Autodesk Inventor part; units mm, degrees
ref_plane "XZ Plane" through (0, 0, 0) normal (0, 1, 0) x (-1, 0, 0)
ref_plane "XY Plane" through (0, 0, 0) normal (0, 0, 1) x (1, 0, 0)
sketch "Sketch2" plane through (0, 0, 0) normal (0, 1, 0) x (-1, 0, 0)
  line L0 (35.5, -4) -> (35.5, 25)
  line L1 (35.5, 25) -> (31.5, 25)
  line L2 (31.5, 25) -> (31.5, 0)
  line L3 (31.5, 0) -> (-31.5, 0)
  line L4 (-31.5, 0) -> (-31.5, 25)
  line L5 (-31.5, 25) -> (-35.5, 25)
  line L6 (-35.5, 25) -> (-35.5, -4)
  line L7 (-35.5, -4) -> (35.5, -4)
  line L8 (0, -9.8) -> (0, 30.8) construction
  line L9 (-49.7, 0) -> (49.7, 0) construction
  point P0 (0, 0)
  dimension "d0" = 4
  dimension "d1" = 25
  dimension "d2" = 71
  dimension "d3" = 4
extrude "Extrusion1" add sketch "Sketch2" along normal blind 3
sketch "Sketch3" plane through (35.5, 0, 25) normal (1, 0, 0) x (0, 0, -1)
  line L0 (0, 0) -> (0, 3) construction
  line L1 (0, 0) -> (0, 3) construction
  line L2 (0, 0.25) -> (-2.7386, 0.25) construction
  circle A0 centre (-2.7386, 0.25) radius 1.25
  circle A1 centre (-2.7386, 0.25) radius 2.75
  line L3 (0, 0) -> (29, 0) construction
  line L4 (0, 3) -> (29, 3) construction
  line L5 (29, 3) -> (0, 3) construction
  line L6 (-2.7386, 3) -> (0, 3) construction
  line L7 (-2.7386, 3) -> (-2.7386, 0.25) construction
  line L8 (-2.7386, 3) -> (0, 3)
  line L9 (0, 0) -> (0, 3)
  point P0 (25, 0)
  dimension "d6" = 2.5
  dimension "d7" = 1.5
extrude "Extrusion2" add sketch "Sketch3" against normal up to surface (4 mm away)
mirror "Mirror1" about plane through (0, 0, 0) normal (1, 0, 0) of "Extrusion2"
fillet "Fillet1" radius 4 4 edges at (-35.5, 1.5, -4) (-31.5, 1.5, 0) (31.5, 1.5, 0) (35.5, 1.5, -4)
equation "\"d3\" = d0"
properties part number "back_support"
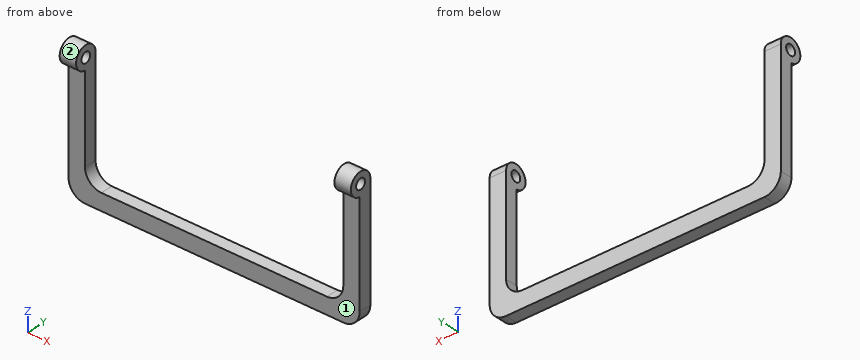
Can you work these out from the model? Positions are in its coordinate system, mm. Face numbers are marked on the shaded views. A direction names the side the tool comes from. Round coordinates to 2 decimals unless told otherwise and drop trailing zeros. Loops run counter-clockwise (first coordinate to the right, second up) from the corner with the lowest first, then second, coordinate; pieces in that order, holes last. Notation, with made-up numbers: M 40,88 L 89,88 A22 ccw 89,107 Z; hole C 89.5,83 d9. An arc over 180 degrees is marked long. Answer in a Markdown table with one row per item.
1. On a 3-axis mill with a long thin cutter (end or side, diameter ignored), from which of +Z, -Z, +X, -X, +Y, -Y can I reach the whole of each face in a straight line? I mean the marked faces 1 and 2. Say none if no direction works.
Established:
| item | result |
|---|---|
| face 1 | -Z, +X, -X, -Y |
| face 2 | +X, -X |
2. I'm going to push flat-ended pins straight in: pin 1 Ø2.5 at (x, y) = (10.5, 1.5) entering from +Z; pin 2 Ø2 at (y, z) = (0.25, 27.74) entering from -X. Where does each tip first touch, or does it pass through?
Established:
| item | result |
|---|---|
| pin 1 | z = 0 |
| pin 2 | through |
3. If we section it at A-A, the plane z = 24: Please give me the cut outline in (x, y), plus the area to 3 significant figures.
Established:
| item | result |
|---|---|
| outline | M -35.5,0 L -31.5,0 L -31.5,3 L -35.5,3 Z; M 31.5,0 L 35.5,0 L 35.5,3 L 31.5,3 Z |
| area | 24.0 mm² |
4. If we section it at B-B, the plane y = -1.75: Please give me the cut outline in (x, z).
Established:
| item | result |
|---|---|
| outline | M -35.5,25.85 L -31.5,25.85 L -31.5,29.63 L -35.5,29.63 Z; M 31.5,25.85 L 35.5,25.85 L 35.5,29.63 L 31.5,29.63 Z |
5. If we section it at C-C, the plane x = -1: Please give me the cut outline in (y, z).
Established:
| item | result |
|---|---|
| outline | M 0,-4 L 3,-4 L 3,0 L 0,0 Z |
6. Please list where these lines run through material, in increasing order: line 1 (X direction, y = 0.5, z = 20.5); line 2 (Z direction, x = 8, y = 2.1); line 3 (Y direction, x = -32, z = -1.5). Write a range as from..to.
Established:
| item | result |
|---|---|
| line 1 | -35.5..-31.5, 31.5..35.5 |
| line 2 | -4..0 |
| line 3 | 0..3 |
7. If we section it at D-D, the plane x = 29: Please give me the cut outline in (y, z), plus the area to 3 significant figures.
Established:
| item | result |
|---|---|
| outline | M 0,-4 L 3,-4 L 3,0.29 L 0,0.29 Z |
| area | 12.9 mm² |
